Read the model definition and answer for the solid it produces. Units are mm, in the model's axes. A direction names the side the tool comes from. Round coordinates to 2 decimals unless told otherwise and drop trailing zeros. Write each loop counter-clockwise with the first axis right and the second up, starting at its lowest first coordinate (ties: lowest second). Pieces come first, ordered by that corner, then holes. Notation, with made-up numbers: (45.25, -24.75) - (79.25, -24.75) arc R17 cw to (79.25, -19.75) - close; hole circle Ø9 at (69, -10.5). An arc over 180 degrees is marked (long way). Use one line per item in the form item = value. Start each with the question number.
1) Each of these flat-tipped pins is pushed along its axis until it touches: pin 1 (3.5 mm diameter, centred on x = 25.25, z = 15.91, fed in from -Y); pin 2 (1 mm diameter, centred on y = -1, z = -15, fed in from +X). Where does it stop, or does it pass through?
2) For faces 5 (the face through (-25.367, -1, -13)), 6 (the face through (2.751, -1, -14)), 7 (the face through (28, -1, 13.406)), determine the directions among +Z, -Z, +X, -X, +Y, -Y from which every point of the face is accessible in a straight line to the end or side of a thin tool.
3) The part is cut by section B-B, the plane z = 1. Give the vertices of the cut face in (x, y), plus the area to 3 significant figures.
4) The part is cut by section A-A, the plane x = 9.5. Give the vertices of the cut face in (y, z).
5) The part is cut by section C-C, the plane y = -1.55. Give the vertices of the cut face in (x, z) (3 decimals), plus the area to 3 significant figures.
6) For a pull along Z with two mould halves and no side action, classify faces 1 (the face through (-22.437, -0.986, -41.376)), 2 (the face through (-21.367, -1, -14)), 3 (the face through (28.751, -1, 16)), 4 (the face through (0, -1, -43.289)) as released by +Z, released by -Z, zero draft, split by the parting line, or undercut.
7) Consider line 1 along X through (y, z) = (-1.05, 10); line 2 along Z through (x, y) = (4.5, -0.05); line 3 along Z through (x, y) = (17.5, -1.5). Determine where each line is inside the solid, lowest interval first. Write a range as from..to.
from build123d import *

# Parameters (mm, degrees)
F1_W     = 56
F1_H     = 5
F1_R     = 1.375
F2_DEPTH = 2
F0_W     = 15
F0_H     = 3
F3_DEPTH = 1
F4_R     = 1.375
F4_W     = 4
F4_H     = 53.2898265516
F5_DEPTH = 2


with BuildPart() as f2:
    # F1 (on Front) → F2 (new body)
    with BuildSketch(Plane.XZ):
        with Locations((0.7514315657, 15.9062612424)):
            Rectangle(F1_W, F1_H)
        with Locations((-23.7485684343, 15.9062612424)):
            Circle(F1_R, mode=Mode.SUBTRACT)
        with Locations((25.2514315657, 15.9062612424)):
            Circle(F1_R, mode=Mode.SUBTRACT)
    extrude(amount=F2_DEPTH)

    # F0 (on Front) → F3 (cut)
    with BuildSketch(Plane.XZ):
        with Locations((0.7514315657, 16.9062612424)):
            Rectangle(F0_W, F0_H)
    extrude(amount=F3_DEPTH, mode=Mode.SUBTRACT)

    # F4 (on Front) → F5 (join)
    with BuildSketch(Plane.XZ):
        with BuildLine():
            Line((-22.1303412057, -39.8835653092), (-25.3667956628, -39.8835653092))
            ThreePointArc((-25.3667956628, -39.8835653092), (-25.4620381693, -43.6096183945), (-21.7485684343, -43.289172991))
            ThreePointArc((-21.7485684343, -43.289172991), (-21.3768601891, -42.579742406), (-21.2485684343, -41.789172991))
            ThreePointArc((-21.2485684343, -41.789172991), (-21.4796955785, -40.7393082548), (-22.1303412057, -39.8835653092))
        make_face()
        with Locations((-23.7485684343, -41.789172991)):
            Circle(F4_R, mode=Mode.SUBTRACT)
        with BuildLine():
            Line((-25.3667956628, 13.6541156098), (-25.3667956628, -39.8835653092))
            ThreePointArc((-25.3667956628, -39.8835653092), (-23.7485684343, -39.289172991), (-22.1303412057, -39.8835653092))
            Line((-22.1303412057, -39.8835653092), (-21.3667956628, -39.8835653092))
            Line((-21.3667956628, -39.8835653092), (-21.3667956628, 9.7079015317))
            Line((-21.3667956628, 9.7079015317), (-21.3667956628, 13.6541156098))
            Line((-21.3667956628, 13.6541156098), (-25.3667956628, 13.6541156098))
        make_face()
        with BuildLine():
            ThreePointArc((-22.1303412057, -39.8835653092), (-23.7485684343, -39.289172991), (-25.3667956628, -39.8835653092))
            Line((-25.3667956628, -39.8835653092), (-22.1303412057, -39.8835653092))
        make_face()
        with BuildLine():
            ThreePointArc((-21.2485684343, -41.789172991), (-21.3768601891, -42.579742406), (-21.7485684343, -43.289172991))
            Line((-21.7485684343, -43.289172991), (-21.3667956628, -43.289172991))
            Line((-21.3667956628, -43.289172991), (23.2514315657, -43.289172991))
            ThreePointArc((23.2514315657, -43.289172991), (22.7514315657, -41.789172991), (23.2514315657, -40.289172991))
            Line((23.2514315657, -40.289172991), (23.2514315657, -39.8835653092))
            Line((23.2514315657, -39.8835653092), (20.2613644372, -39.8835653092))
            Line((20.2613644372, -39.8835653092), (2.7514315657, -39.8835653092))
            Line((2.7514315657, -39.8835653092), (-1.2485684343, -39.8835653092))
            Line((-1.2485684343, -39.8835653092), (-21.3667956628, -39.8835653092))
            Line((-21.3667956628, -39.8835653092), (-22.1303412057, -39.8835653092))
            ThreePointArc((-22.1303412057, -39.8835653092), (-21.4796955785, -40.7393082548), (-21.2485684343, -41.789172991))
        make_face()
        with BuildLine():
            Line((23.3217352043, -43.3785980293), (23.2514315657, -43.289172991))
            ThreePointArc((23.2514315657, -43.289172991), (23.2860747069, -43.3342854197), (23.3217352043, -43.3785980293))
        make_face()
        with BuildLine():
            ThreePointArc((23.2514315657, -40.289172991), (22.7514315657, -41.789172991), (23.2514315657, -43.289172991))
            Line((23.2514315657, -43.289172991), (23.2514315657, -40.289172991))
        make_face()
        with BuildLine():
            Line((23.2514315657, -40.289172991), (23.2514315657, -43.289172991))
            Line((23.2514315657, -43.289172991), (23.3217352043, -43.3785980293))
            ThreePointArc((23.3217352043, -43.3785980293), (26.0957535115, -44.1422816693), (27.7514315657, -41.789172991))
            ThreePointArc((27.7514315657, -41.789172991), (27.6231398109, -40.998603576), (27.2514315657, -40.289172991))
            Line((27.2514315657, -40.289172991), (23.2514315657, -40.289172991))
        make_face()
        with Locations((25.2514315657, -41.789172991)):
            Circle(F4_R, mode=Mode.SUBTRACT)
        with Locations((0.7514315657, -13.2386520334)):
            Rectangle(F4_W, F4_H)
        with BuildLine():
            Line((23.2514315657, -39.8835653092), (23.2514315657, -40.289172991))
            ThreePointArc((23.2514315657, -40.289172991), (25.2514315657, -39.289172991), (27.2514315657, -40.289172991))
            Line((27.2514315657, -40.289172991), (27.2514315657, 13.6541156098))
            Line((27.2514315657, 13.6541156098), (23.2514315657, 13.6541156098))
            Line((23.2514315657, 13.6541156098), (23.2514315657, -35.9635577695))
            Line((23.2514315657, -35.9635577695), (23.2514315657, -39.8835653092))
        make_face()
        with BuildLine():
            ThreePointArc((27.2514315657, -40.289172991), (25.2514315657, -39.289172991), (23.2514315657, -40.289172991))
            Line((23.2514315657, -40.289172991), (27.2514315657, -40.289172991))
        make_face()
    extrude(amount=F5_DEPTH)


solid = f2.part
Geometry results:
q1.pin_1 = -2
q1.pin_2 = 27.25
q2.face_5 = -X, +Y, -Y
q2.face_6 = +Y, -Y
q2.face_7 = +X, +Y, -Y
q3.outline = (-25.37, -2) - (-21.37, -2) - (-21.37, 0) - (-25.37, 0) - close; (-1.25, -2) - (2.75, -2) - (2.75, 0) - (-1.25, 0) - close; (23.25, -2) - (27.25, -2) - (27.25, 0) - (23.25, 0) - close
q3.area = 24.0 mm2
q4.outline = (-2, -43.29) - (0, -43.29) - (0, -39.88) - (-2, -39.88) - close; (-2, 13.41) - (0, 13.41) - (0, 18.41) - (-2, 18.41) - close
q5.outline = (-27.249, 13.406) - (-25.367, 13.406) - (-25.367, -39.884) arc R2.5 ccw (long way) to (-21.749, -43.289) - (23.251, -43.289) arc R2.5 ccw to (27.251, -40.289) - (27.251, 13.406) - (28.751, 13.406) - (28.751, 18.406) - (-27.249, 18.406) - close; hole circle Ø2.75 at (-23.749, -41.789); hole circle Ø2.75 at (-23.749, 15.906); hole (-21.367, -39.884) - (-1.249, -39.884) - (-1.249, 13.406) - (-21.367, 13.406) - close; hole (2.751, -39.884) - (23.251, -39.884) - (23.251, 13.406) - (2.751, 13.406) - close; hole circle Ø2.75 at (25.251, -41.789); hole circle Ø2.75 at (25.251, 15.906)
q5.area = 1,080 mm2
q6.face_1 = undercut
q6.face_2 = undercut
q6.face_3 = zero draft
q6.face_4 = released by -Z
q7.line_1 = -25.37..-21.37, -1.25..2.75, 23.25..27.25
q7.line_2 = -43.29..-39.88, 13.41..15.41
q7.line_3 = -43.29..-39.88, 13.41..18.41
